```python
from build123d import *

# Parameters (mm, degrees)
F1_DEPTH = 40
F2_R     = 4.25
F3_DEPTH = 25
F4_R     = 15
F5_R     = 5
F6_W     = 56.803
F6_H     = 10.5
F7_DEPTH = 4
F8_DEPTH = 5


with BuildPart() as f1:
    # F0 (on Front) → F1 (new body)
    with BuildSketch(Plane.XZ):
        Polygon((-45, 0), (0, 0), (0, 5), (-45, 5), (-45, 70), (-45, 75), (-125, 75), (-125, 70), (-50, 70), (-50, 0), align=None)
    extrude(amount=F1_DEPTH)

    # F2 (on face) → F3 (cut)
    with BuildSketch(Plane(origin=(0, 0, 0), x_dir=(1, 0, 0), z_dir=(0, 0, -1))):
        with Locations((-17, 20)):
            Circle(F2_R)
    extrude(amount=-F3_DEPTH, mode=Mode.SUBTRACT)

    # F4
    f4_edges = [f1.edges().sort_by_distance(p)[0] for p in [
        (-45, -20, 5),
        (-50, -20, 70),
    ]]
    fillet(f4_edges, radius=F4_R)

    # F5
    f5_edges = [f1.edges().sort_by_distance(p)[0] for p in [
        (-45, -20, 75),
        (-50, -20, 0),
    ]]
    fillet(f5_edges, radius=F5_R)

    # F6 (on face) → F7 (cut)
    with BuildSketch(Plane.XZ.offset(40)):
        with Locations((-28.4015, 5.25)):
            Rectangle(F6_W, F6_H)
    extrude(amount=-F7_DEPTH, mode=Mode.SUBTRACT)

    # F8 (add): a face of the model
    f8_faces = [f1.faces().sort_by_distance(p)[0] for p in [
        (-125, -20, 72.5),
    ]]
    extrude(f8_faces, amount=F8_DEPTH)


solid = f1.part
```
Could you check a few things on this model? Use its own coordinates, in mm. A direction names the side the tool comes from. Give positions to 0.01 mm unless a question says otherwise; leave off trailing zeros. Order: outer loops, then holes, each group sorted by start corner. A loop starts at its lowest first (then second) coordinate and runs counter-clockwise, first axis right, second up.
Q1. Suppose I cut it at A-A, the plane x = -17. Write out the boundary of the cut face in (y, z).
Q2. Suppose I cut it at B-B, the plane y = -20. Write out the boundary of the cut face in (x, z).
Q3. For faces 1 (the flat face through (-45, -20, 45)), 2 (the flat face through (-50, -20, 30)), 3 (the flat face through (-46, -38, 10.5)), which set-ups out of +Z, -Z, +X, -X, +Y, -Y let a thin tool reach every point of the face, with its end or its side?
Q4. We'd pull the mould along Y, two halves only. Please class faces 4 (the flat face through (-31, -36, 4)), 5 (the cylindrical face through (-15.04, -16.23, 2.46)), 6 (the flat face through (-45.4, 0, 46)): +Y half, -Y half, draft (parallel to the pull), parting line (faces both ways), or undercut.
Q5. If I drill on line 1 along Y through (x, z) = (-17, 3.2); line 2 along Z through (x, y) = (-118, -6); line 3 along X through (y, z) = (-20, 1.2), over which ranges is the centre line in solid material (lowest first)?
Q6. Suppose I cut it at D-D, the plane x = -97.5. Write out the boundary of the cut face in (y, z), and give its area (3 significant figures).
Q7. Suppose I cut it at C-C, the plane y = -9.5. Write out the boundary of the cut face in (x, z).
Q8. I'm going to push flat-ended pins straight in: P1, Ø12, axis at y = -9.5, z = 30.5, coming from the -X side; P2, Ø7.5, axis at x = -17, y = -20, coming from the -Z side; P3, Ø10, axis at x = -42.5, z = 30, coming from the -Y side; P4, Ø15, axis at x = -8.5, y = -12.5, coming from the +Z side. Where does each tip first touch, or does it pass through?
Solution:
1. outline: (-36, 0) - (-24.25, 0) - (-24.25, 5) - (-36, 5) - close; (-15.75, 0) - (0, 0) - (0, 5) - (-15.75, 5) - close
2. outline: (-130, 70) - (-65, 70) arc R15 cw to (-50, 55) - (-50, 5) arc R5 ccw to (-45, 0) - (-21.25, 0) - (-21.25, 5) - (-30, 5) arc R15 cw to (-45, 20) - (-45, 70) arc R5 ccw to (-50, 75) - (-130, 75) - close; (-12.75, 0) - (0, 0) - (0, 5) - (-12.75, 5) - close
3. face 1: +Z, +X, +Y, -Y
3. face 2: -Z, -X, +Y, -Y
3. face 3: -Z, +X, -X, -Y
4. face 4: -Y half
4. face 5: undercut
4. face 6: +Y half
5. line 1: y = -36 to -24.25, -15.75 to 0
5. line 2: z = 70 to 75
5. line 3: x = -48.25 to -21.25, -12.75 to 0
6. outline: (-40, 70) - (0, 70) - (0, 75) - (-40, 75) - close
6. area: 200 mm2
7. outline: (-130, 70) - (-65, 70) arc R15 cw to (-50, 55) - (-50, 5) arc R5 ccw to (-45, 0) - (0, 0) - (0, 5) - (-30, 5) arc R15 cw to (-45, 20) - (-45, 70) arc R5 ccw to (-50, 75) - (-130, 75) - close
8. P1: stops at x = -50
8. P2: passes through
8. P3: stops at y = -40
8. P4: stops at z = 5
